from build123d import *

# Parameters (mm, degrees)
F0_W     = 100
F0_H     = 24
F1_DEPTH = 9
F2_R     = 5
F3_W     = 35
F3_H     = 10
F4_W     = 35
F4_H     = 10
F5_DEPTH = 2
F6_R     = 3
F7_W     = 35
F7_H     = 10
F8_DEPTH = 2
F9_R     = 3
F10_SIZE = 1


with BuildPart() as f1:
    # F0 (on Top) → F1 (new body)
    with BuildSketch(Plane.XY):
        with Locations((0, 12)):
            Rectangle(F0_W, F0_H)
    extrude(amount=F1_DEPTH)

    # F2
    f2_edges = [f1.edges().sort_by_distance(p)[0] for p in [
        (-50, 0, 4.5),
        (50, 0, 4.5),
    ]]
    fillet(f2_edges, radius=F2_R)

    # F3 (on face) + F4 (on face) → F5 (cut)
    with BuildSketch(Plane.XY.offset(9)):
        with Locations((-27.5, 12)):
            Rectangle(F3_W, F3_H)
    with BuildSketch(Plane.XY.offset(9)):
        with Locations((27.5, 12)):
            Rectangle(F4_W, F4_H)
    extrude(amount=-F5_DEPTH, mode=Mode.SUBTRACT)

    # F6
    f6_edges = [f1.edges().sort_by_distance(p)[0] for p in [
        (-45, 7, 8),
        (-45, 17, 8),
        (-10, 17, 8),
        (10, 7, 8),
        (-10, 7, 8),
        (45, 7, 8),
        (45, 17, 8),
        (10, 17, 8),
    ]]
    fillet(f6_edges, radius=F6_R)

    # F7 (on face) → F8 (cut)
    with BuildSketch(Plane(origin=(0, 0, 0), x_dir=(1, 0, 0), z_dir=(0, 0, -1))):
        with Locations((-27.5, -12)):
            Rectangle(F7_W, F7_H)
        with Locations((27.5, -12)):
            Rectangle(F7_W, F7_H)
    extrude(amount=-F8_DEPTH, mode=Mode.SUBTRACT)

    # F9
    f9_edges = [f1.edges().sort_by_distance(p)[0] for p in [
        (45, 17, 1),
        (-10, 17, 1),
        (10, 17, 1),
        (-45, 17, 1),
        (10, 7, 1),
        (-45, 7, 1),
        (-10, 7, 1),
        (45, 7, 1),
    ]]
    fillet(f9_edges, radius=F9_R)

    # F10
    f10_edges = [f1.edges().sort_by_distance(p)[0] for p in [
        (0, 0, 9),
        (0, 0, 0),
    ]]
    chamfer(f10_edges, length=F10_SIZE)


solid = f1.part
Could you check a few things on this model? Use its own coordinates, in mm. A direction names the side the tool comes from. Give positions to 0.01 mm unless a question says otherwise; leave off trailing zeros. Loops run counter-clockwise (first coordinate to the right, second up) from the corner with the lowest first, then second, coordinate; pieces in that order, holes last. Notation, with made-up numbers: M -10,23 L 27,23 A31 cw 27,58 Z; hole C 23,5 d11. An arc over 180 degrees is marked long. Answer as a JSON object with one key per item and string values.
Q1. If we mould it in two halves opening along Y, with no side actions, what happens to faces 3 (the flat face through (-1, 13, 0)), 4 (the conical face through (-48.063, 2.004, 0.285)), 5 (the flat face through (27, 12, 2))? For each: pulls with the +Y half, pulls with the -Y half, needs draft (parallel to the pull), parting line crosses it, or undercut.
Values found:
{"face 3": "needs draft", "face 4": "pulls with the -Y half", "face 5": "undercut"}
Q2. If I drill on probe 1 along Y at (x, z) = (24.5, 1.75); probe 2 along Y at (x, z) = (28.5, 0.5); probe 3 along Z at (x, y) = (38, 15.5), over which ranges is the centre line in solid material (lowest first)? Write a range as [from, to].
Values found:
{"probe 1": "y = [0, 7], [17, 24]", "probe 2": "y = [0.5, 7], [17, 24]", "probe 3": "z = [2, 7]"}
Q3. Suppose I cut it at A-A, the plane x = -23.5. List the corners of the cut face in (y, z) for me, plus the area to 3 significant figures.
Values found:
{"outline": "M 0,1 L 1,0 L 7,0 L 7,2 L 17,2 L 17,0 L 24,0 L 24,9 L 17,9 L 17,7 L 7,7 L 7,9 L 1,9 L 0,8 Z", "area": "175 mm²"}
Q4. Suppose I cut it at C-C, the plane y = 8.25. List the corners of the cut face in (x, z) for me.
Values found:
{"outline": "M -50,1 L -49,0 L -44.44,0 L -44.44,2 L -10.56,2 L -10.56,0 L 10.56,0 L 10.56,2 L 44.44,2 L 44.44,0 L 49,0 L 50,1 L 50,8 L 49,9 L 44.44,9 L 44.44,7 L 10.56,7 L 10.56,9 L -10.56,9 L -10.56,7 L -44.44,7 L -44.44,9 L -49,9 L -50,8 Z"}
Q5. Suppose I cut it at B-B, the plane y = 12. List the corners of the cut face in (x, z) for me.
Values found:
{"outline": "M -50,1 L -49,0 L -45,0 L -45,2 L -10,2 L -10,0 L 10,0 L 10,2 L 45,2 L 45,0 L 49,0 L 50,1 L 50,8 L 49,9 L 45,9 L 45,7 L 10,7 L 10,9 L -10,9 L -10,7 L -45,7 L -45,9 L -49,9 L -50,8 Z"}
Q6. For faces 1 (the flat face through (27, 7, 1)), 2 (the cylindrical face through (-44.1, 7.86, 7.99)), which set-ups out of +Z, -Z, +X, -X, +Y, -Y let a thin tool reach every point of the face, with its end or its side?
Values found:
{"face 1": "-Z", "face 2": "+Z"}
Q7. For P1, Ø0.6, axis at x = -31, z = 8.5, coming from the -Y side; P2, Ø3, axis at x = 24, y = 10, coming from the +Z side; P3, Ø5, axis at x = 36, y = 11.5, coming from the -Z side, each with a flat end and sliding along its axis, tell me the tip position at first contact or that it passes through.
Values found:
{"P1": "stops at y = 0.2", "P2": "stops at z = 7", "P3": "stops at z = 2"}
